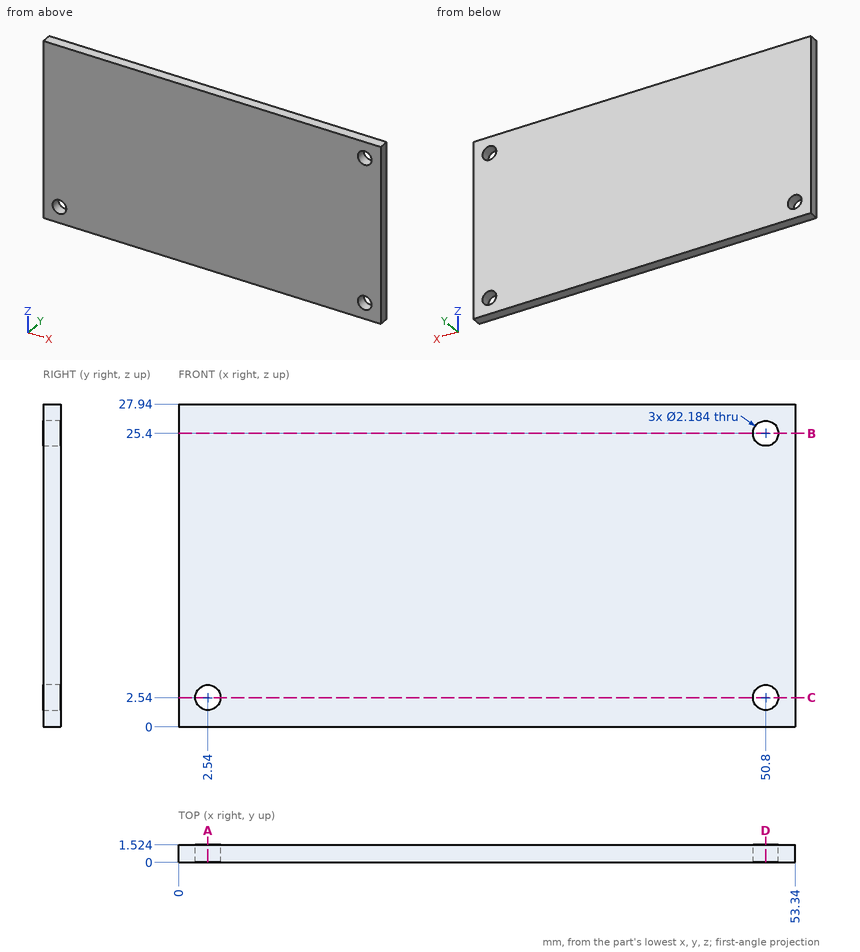
Verification items for this drawing (mm, ordinates from the low corner). Round coordinates to 2 decimals unless told otherwise and drop trailing zeros. Order: outer loops, then holes, each group sorted by start corner. A loop starts at its lowest first (then second) coordinate and runs counter-clockwise, first axis right, second up. Notation, with made-up numbers: (17, -32.5) - (60, -32.5) arc R27 ccw to (60, -4.5) - close; hole circle Ø8 at (10, -6). An arc over 180 degrees is marked (long way). Use CSV: the item, a comma, the result in double quotes.
(1) Section check A-A on x = 2.54. Record the boundary of the cut face in (y, z).
Entries:
outline,"(0, 0) - (1.52, 0) - (1.52, 1.45) - (0, 1.45) - close; (0, 3.63) - (1.52, 3.63) - (1.52, 27.94) - (0, 27.94) - close"
(2) Section check C-C on z = 2.54. Record the boundary of the cut face in (x, y).
Entries:
outline,"(0, 0) - (1.45, 0) - (1.45, 1.52) - (0, 1.52) - close; (3.63, 0) - (49.71, 0) - (49.71, 1.52) - (3.63, 1.52) - close; (51.89, 0) - (53.34, 0) - (53.34, 1.52) - (51.89, 1.52) - close"
(3) Thickness scan on probe 1 along X at (y, z) = (1.2, 2.5); probe 2 along Z at (x, y) = (50, 1.2) (1 decimal). Record the ranges inside material, lowest first. Write a range as from..to.
Entries:
probe 1,"0..1.45, 3.63..49.71, 51.89..53.34"
probe 2,"0..1.8, 3.3..24.7, 26.1..27.9"
(4) Section check D-D on x = 50.8. Record the boundary of the cut face in (y, z).
Entries:
outline,"(0, 0) - (1.52, 0) - (1.52, 1.45) - (0, 1.45) - close; (0, 3.63) - (1.52, 3.63) - (1.52, 24.31) - (0, 24.31) - close; (0, 26.49) - (1.52, 26.49) - (1.52, 27.94) - (0, 27.94) - close"
(5) Gauge pin test, flat end, axial feed: pin 1 Ø2.5 at (x, z) = (2.54, 2.54) entering from +Y. Record the tip position at first contact, or that the pin passes through.
Entries:
pin 1,"y = 1.52"
(6) Section check B-B on z = 25.4. Record the boundary of the cut face in (x, y).
Entries:
outline,"(0, 0) - (49.71, 0) - (49.71, 1.52) - (0, 1.52) - close; (51.89, 0) - (53.34, 0) - (53.34, 1.52) - (51.89, 1.52) - close"
